Geometry check sheet. Reference: the model listing, model coordinates, mm. A direction names the side the tool comes from. Coordinates: 2 decimals unless noted, no trailing zeros. Order: outer loops, then holes, each group sorted by start corner. A loop starts at its lowest first (then second) coordinate and runs counter-clockwise, first axis right, second up. Notation, with made-up numbers: (0, 2.25) - (26, 2.25) arc R20 cw to (26, 39.25) - close; hole circle Ø3 at (-19, 6.25). An arc over 180 degrees is marked (long way). Return JSON: item names as keys, results as strings. Group by question number.
Item 1: Section check B-B on x = -2. Give the number of separate pieces and of enclosed holes in the cut face, then the cut area to 3 significant figures.
Item 2: Section check A-A on z = 50. Enter the section's corners in (x, y), then the cut area to 3 significant figures.
Item 3: Gauge pin test, flat ends, axial feed: pin 1 (8 mm diameter, centred on x = 0, z = 150, fed in from -Y); pin 2 (19.5 mm diameter, centred on x = 0, z = 150, fed in from +Y); pin 3 (7.5 mm diameter, centred on x = -18, z = 152.5, fed in from -Y); pin 4 (13.5 mm diameter, centred on x = 0, z = 50, fed in from +Y). Record the tip position at first contact, or that the pin passes through.
Item 4: Tool access check on faces 4 (the cylindrical face through (39.115, 10.21, 184.46)), 5 (the cylindrical face through (-20.828, -7.525, 10.14)), 6 (the flat face through (-18, -18.5, 45)), 7 (the flat face through (-50, 0, 99)), 8 (the cylindrical face through (-34.79, 9.73, 38.5)). Record the directions out of +Z, -Z, +X, -X, +Y, -Y that give a thin tool (end or side, any length) a straight path to the whole face; none if there is none.
Item 5: Scan lines: probe 1 along Z at (x, y) = (-17.5, 16.5); probe 2 along X at (y, z) = (-14, 150); probe 3 along Z at (x, y) = (-17, -13). Record each from-to range of solid material in increasing order.
Item 6: Draft check along Z on faces 1 (the flat face through (-1, -25, 99)), 2 (the conical face through (-35.715, -7.061, 15.094)), 3 (the flat face through (0, -9.5, 45)). Enter one of: pulls with the +Z half, pulls with the -Z half, needs draft (parallel to the pull), parting line crosses it, or undercut.
from build123d import *

# Parameters (mm, degrees)
SKIZZE1_W                                           = 100
SKIZZE1_H                                           = 50
AUFSATZ_LINEAR_AUSTRAGEN1_DEPTH                     = 200
STIRNSENKUNG_F_R_M8_SENKSCHRAUBE_KOPF_B_D           = 9
STIRNSENKUNG_F_R_M8_SENKSCHRAUBE_KOPF_B_CBORE_D     = 15
STIRNSENKUNG_F_R_M8_SENKSCHRAUBE_KOPF_B_CBORE_DEPTH = 34.5
STIRNSENKUNG_F_R_M8_SENKSCHRAUBE_KO_2_D             = 9
STIRNSENKUNG_F_R_M8_SENKSCHRAUBE_KO_2_DEPTH         = 50
STIRNSENKUNG_F_R_M8_SENKSCHRAUBE_KO_2_CBORE_D       = 15
STIRNSENKUNG_F_R_M8_SENKSCHRAUBE_KO_2_CBORE_DEPTH   = 6.5
SPIEGELN4_COPY_1_D                                  = 9
SPIEGELN4_COPY_1_CBORE_D                            = 15
SPIEGELN4_COPY_1_CBORE_DEPTH                        = 34.5
SPIEGELN4_COPY_2_D                                  = 9
SPIEGELN4_COPY_2_DEPTH                              = 50
SPIEGELN4_COPY_2_CBORE_D                            = 15
SPIEGELN4_COPY_2_CBORE_DEPTH                        = 6.5
KERNLOCH_F_R_M8_HELICOIL3_D                         = 8.3
KERNLOCH_F_R_M8_HELICOIL3_DEPTH                     = 20
KERNLOCH_F_R_M8_HELICOIL3_TIP                       = 2.493571569
KERNLOCH_F_R_M8_HELICOIL4_D                         = 8.3
KERNLOCH_F_R_M8_HELICOIL4_DEPTH                     = 20
KERNLOCH_F_R_M8_HELICOIL4_TIP                       = 2.493571569


# Read off the part's stored shape, not the designer's step: Kernloch für M8 Helicoil2
with BuildPart() as part:
    # Skizze1 → Aufsatz-Linear austragen1 (new body)
    with BuildSketch(Plane.XY):
        Rectangle(SKIZZE1_W, SKIZZE1_H)
    extrude(amount=AUFSATZ_LINEAR_AUSTRAGEN1_DEPTH)

    # Stirnsenkung f_r M8 Senkschraube _Kopf B (through all)
    with Locations(Plane(origin=(0, 25, 0), x_dir=(1, 0, 0), z_dir=(0, 1, 0))):
        with Locations((0, -150)):
            stirnsenkung_f_r_m8_senkschraube_kopf_b = CounterBoreHole(STIRNSENKUNG_F_R_M8_SENKSCHRAUBE_KOPF_B_D / 2, STIRNSENKUNG_F_R_M8_SENKSCHRAUBE_KOPF_B_CBORE_D / 2, STIRNSENKUNG_F_R_M8_SENKSCHRAUBE_KOPF_B_CBORE_DEPTH)

    # Stirnsenkung f_r M8 Senkschraube _Ko 2
    with Locations(Plane(origin=(0, -25, 0), x_dir=(-1, 0, 0), z_dir=(0, -1, 0))):
        with Locations((0, -150)):
            stirnsenkung_f_r_m8_senkschraube_ko_2 = CounterBoreHole(STIRNSENKUNG_F_R_M8_SENKSCHRAUBE_KO_2_D / 2, STIRNSENKUNG_F_R_M8_SENKSCHRAUBE_KO_2_CBORE_D / 2, STIRNSENKUNG_F_R_M8_SENKSCHRAUBE_KO_2_CBORE_DEPTH, depth=STIRNSENKUNG_F_R_M8_SENKSCHRAUBE_KO_2_DEPTH)

    # Spiegeln1: Stirnsenkung f_r M8 Senkschraube _Kopf B, Stirnsenkung f_r M8 Senkschraube _Ko 2 across plane
    add(stirnsenkung_f_r_m8_senkschraube_kopf_b.mirror(Plane.XY.offset(100)), mode=Mode.SUBTRACT)
    add(stirnsenkung_f_r_m8_senkschraube_ko_2.mirror(Plane.XY.offset(100)), mode=Mode.SUBTRACT)

    # Skizze10 → Kernloch für M8 Helicoil1 (revolve, cut)
    with BuildSketch(Plane(origin=(-35, 25, 185), x_dir=(0, 0, 1), z_dir=(1, 0, 0))):
        Polygon((0, 0), (0, 32.493571569), (4.15, 30), (4.15, 0), align=None)
    kernloch_f_r_m8_helicoil1 = revolve(axis=Axis((-35, 31.35, 185), (0, -1, 0)), mode=Mode.SUBTRACT)

    # Spiegeln2: Kernloch für M8 Helicoil1 across plane
    add(kernloch_f_r_m8_helicoil1.mirror(Plane(origin=(0, 0, 0), x_dir=(0, 0, 1), z_dir=(1, 0, 0))), mode=Mode.SUBTRACT)

    # Spiegeln3: Kernloch für M8 Helicoil1 across plane
    add(kernloch_f_r_m8_helicoil1.mirror(Plane.XY.offset(100)), mode=Mode.SUBTRACT)

    # Spiegeln3 copy 1 sketch → Spiegeln3 copy 1 (revolve, cut)
    with BuildSketch(Plane(origin=(35, 25, 15), x_dir=(0, 0, -1), z_dir=(-1, 0, 0))):
        Polygon((0, 0), (0, 32.493571569), (4.15, 30), (4.15, 0), align=None)
    revolve(axis=Axis((35, 31.35, 15), (0, -1, 0)), mode=Mode.SUBTRACT)

    # Kernloch für M8 Helicoil2 outline → Kernloch für M8 Helicoil2 (revolve, cut)
    with BuildSketch(Plane(origin=(0, 7.5, 35), x_dir=(0, 1, 0), z_dir=(0, 0, -1))):
        Polygon((4.15, -20), (0, -17.506428431), (0, -50), (4.15, -50), align=None)
    revolve(axis=Axis((0, 7.5, 35), (1, 0, 0)), mode=Mode.SUBTRACT)

    # Kernloch f_r M8 Helicoil2 2 outline → Kernloch f_r M8 Helicoil2 2 (revolve, cut)
    with BuildSketch(Plane(origin=(0, 7.5, 165), x_dir=(0, 1, 0), z_dir=(0, 0, -1))):
        Polygon((4.15, -20), (0, -17.506428431), (0, -50), (4.15, -50), align=None)
    revolve(axis=Axis((0, 7.5, 165), (1, 0, 0)), mode=Mode.SUBTRACT)

    # Spiegeln4: Stirnsenkung f_r M8 Senkschraube _Kopf B, Stirnsenkung f_r M8 Senkschraube _Ko 2 across plane
    add(stirnsenkung_f_r_m8_senkschraube_kopf_b.mirror(Plane(origin=(-8.75, 0, 0), x_dir=(0, 0, 1), z_dir=(1, 0, 0))), mode=Mode.SUBTRACT)
    add(stirnsenkung_f_r_m8_senkschraube_ko_2.mirror(Plane(origin=(-8.75, 0, 0), x_dir=(0, 0, 1), z_dir=(1, 0, 0))), mode=Mode.SUBTRACT)

    # Spiegeln4 copy 1 (through all)
    with Locations(Plane(origin=(-17.5, 25, 200), x_dir=(-1, 0, 0), z_dir=(0, 1, 0))):
        with Locations((0, -150)):
            CounterBoreHole(SPIEGELN4_COPY_1_D / 2, SPIEGELN4_COPY_1_CBORE_D / 2, SPIEGELN4_COPY_1_CBORE_DEPTH)

    # Spiegeln4 copy 2
    with Locations(Plane(origin=(-17.5, -25, 200), x_dir=(1, 0, 0), z_dir=(0, -1, 0))):
        with Locations((0, -150)):
            CounterBoreHole(SPIEGELN4_COPY_2_D / 2, SPIEGELN4_COPY_2_CBORE_D / 2, SPIEGELN4_COPY_2_CBORE_DEPTH, depth=SPIEGELN4_COPY_2_DEPTH)

    # Kernloch für M8 Helicoil3
    with Locations(Plane.XY.offset(200)):
        with Locations((4.444e-06, 5)):
            Hole(KERNLOCH_F_R_M8_HELICOIL3_D / 2, depth=KERNLOCH_F_R_M8_HELICOIL3_DEPTH)
            with Locations((0, 0, -(KERNLOCH_F_R_M8_HELICOIL3_DEPTH + KERNLOCH_F_R_M8_HELICOIL3_TIP / 2))):  # 118° drill point
                Cone(0, KERNLOCH_F_R_M8_HELICOIL3_D / 2, KERNLOCH_F_R_M8_HELICOIL3_TIP, mode=Mode.SUBTRACT)

    # Kernloch für M8 Helicoil4
    with Locations(Plane(origin=(0, 0, 0), x_dir=(-1, 0, 0), z_dir=(0, 0, -1))):
        with Locations((17.534722222, -5)):
            Hole(KERNLOCH_F_R_M8_HELICOIL4_D / 2, depth=KERNLOCH_F_R_M8_HELICOIL4_DEPTH)
            with Locations((0, 0, -(KERNLOCH_F_R_M8_HELICOIL4_DEPTH + KERNLOCH_F_R_M8_HELICOIL4_TIP / 2))):  # 118° drill point
                Cone(0, KERNLOCH_F_R_M8_HELICOIL4_D / 2, KERNLOCH_F_R_M8_HELICOIL4_TIP, mode=Mode.SUBTRACT)


solid = part.part
Computed:
{
 "1": {"separate pieces": "3", "enclosed holes": "0", "area": "8,520 mm²"},
 "2": {"outline": "(-50, -25) - (-25, -25) - (-25, -18.5) - (-22, -18.5) - (-22, -9.5) - (-25, -9.5) - (-25, 25) - (-50, 25) - close; (-13, -18.5) - (-10, -18.5) - (-10, -25) - (-7.5, -25) - (-7.5, -18.5) - (-4.5, -18.5) - (-4.5, -9.5) - (-7.5, -9.5) - (-7.5, 25) - (-10, 25) - (-10, -9.5) - (-13, -9.5) - close; (4.5, -18.5) - (7.5, -18.5) - (7.5, -25) - (50, -25) - (50, 25) - (7.5, 25) - (7.5, -9.5) - (4.5, -9.5) - close", "area": "3,610 mm²"},
 "3": {"pin 1": "passes through", "pin 2": "stops at y = 25", "pin 3": "stops at y = -18.5", "pin 4": "stops at y = -9.5"},
 "4": {"face 4": "+Y", "face 5": "-Z", "face 6": "-Y", "face 7": "+Z, -Z, -X, +Y, -Y", "face 8": "-X"},
 "5": {"probe 1": "z = 0 to 42.5, 57.5 to 142.5, 157.5 to 200", "probe 2": "x = -50 to -22, -13 to -4.5, 4.5 to 50", "probe 3": "z = 0 to 45.53, 54.47 to 145.53, 154.47 to 200"},
 "6": {"face 1": "needs draft", "face 2": "undercut", "face 3": "undercut"}
}
